Read the model definition and answer for the solid it produces. Units are mm, in the model's axes. Face numbers are marked on the shaded views. Round coordinates to 2 decimals unless told otherwise and drop trailing zeros. Order: outer loops, then holes, each group sorted by start corner. A loop starts at its lowest first (then second) coordinate and runs counter-clockwise, first axis right, second up. Notation, with made-up numbers: (12, 80.5) -> (54, 80.5) arc R13 cw to (54, 89.5) -> close; hole circle Ø7 at (14.25, 28). An arc over 180 degrees is marked (long way). Answer as a JSON object with one key per item and string values. Group by question number.
Item 1: Given P1, Ø4, axis at x = -99, z = 11.5, coming from the +Y side; P2, Ø12, axis at x = 26.5, z = -10, coming from the +Y side; P3, Ø4, axis at x = -99.5, y = 18.5, coming from the +Z side; P4, Ø8, axis at x = -56.5, y = 8, coming from the -Z side, each flat-ended and moving along its own axis, determine where each tip first touches the part or whether it passes through.
Item 2: Section A-A, the plane y = 7 is taken. Write down the section's boundary in (x, z).
Item 3: Consider probe 1 along Z at (x, y) = (-62.5, 6); probe 2 along Y at (x, z) = (50, -9); probe 3 along X at (y, z) = (23.5, -11.5). Determine where each line is inside the solid, lowest interval first. Write a range as from..to.
Item 4: Section D-D, the plane y = 23 is taken. Count the separate pieces of the cut face and the enclosed holes in it, plus the area to 3 significant figures.
Item 5: Section C-C, the plane y = 41.5 is taken. Write down the section's boundary in (x, z).
Item 6: Section B-B, the plane x = -50.5 is taken. Write down the section's boundary in (y, z).
Item 7: The mould has two halves that part along X. Classify the marked faces 1, 2, 3 and 4: pulls with the +X half, pulls with the -X half, needs draft (parallel to the pull), parting line crosses it, or undercut.
from build123d import *

# Parameters (mm, degrees)
ESQUISSE1_W                 = 50
ESQUISSE1_H                 = 50
ESQUISSE1_W_2               = 140
ESQUISSE1_H_2               = 12
BOSS_EXTRU_2_DEPTH          = 12
BOSS_EXTRU_3_DEPTH          = 30
ESQUISSE3_R                 = 4.25
ENL_V_MAT_EXTRU_1_DEPTH     = 110.627399686
ESQUISSE4_R                 = 2.5
ENL_V_MAT_EXTRU_2_DEPTH     = 8
CHANFREIN2_SIZE             = 10
CONG_1_START                = 0.042620229
CONG_1_DEPTH                = 12
BOSS_EXTRU_4_DEPTH          = 40
ENL_V_START                 = -12
ENL_V_MAT_EXTRU_3_OUTLINE_R = 2.5
ENL_V_MAT_EXTRU_3_DEPTH     = 52
ESQUISSE8_R                 = 2.5
ENL_V_MAT_EXTRU_4_DEPTH     = 12


with BuildPart() as part:
    # Esquisse1 → Boss.-Extru.2 (new body)
    with BuildSketch(Plane(origin=(0, 0, 0), x_dir=(1, 0, 0), z_dir=(0, 1, 0))):
        with Locations((69.411764706, -6.042620229)):
            Rectangle(ESQUISSE1_W, ESQUISSE1_H)
        with Locations((-25.588235294, -6.042620229)):
            Rectangle(ESQUISSE1_W_2, ESQUISSE1_H_2)
    extrude(amount=BOSS_EXTRU_2_DEPTH)

    # Esquisse2 → Boss.-Extru.3 (add)
    with BuildSketch(Plane(origin=(0, 0, 0), x_dir=(1, 0, 0), z_dir=(0, 1, 0))):
        Polygon((-95.588235294, -0.042620229), (-95.588235294, 13.957379771), (-103.588235294, 13.957379771), (-103.588235294, -26.042620229), (-95.588235294, -26.042620229), (-95.588235294, -12.042620229), align=None)
    extrude(amount=BOSS_EXTRU_3_DEPTH)

    # Esquisse3 → Enlèv. mat.-Extru.1 (cut, through all)
    with BuildSketch(Plane(origin=(0, 12, 0), x_dir=(1, 0, 0), z_dir=(0, 1, 0))):
        with Locations(Location((69.411764706, -6.042620229, 0), (0, 0, 270))):
            Circle(ESQUISSE3_R)
    extrude(amount=-ENL_V_MAT_EXTRU_1_DEPTH, mode=Mode.SUBTRACT)

    # Esquisse4 → Enlèv. mat.-Extru.2 (cut)
    with BuildSketch(Plane.ZY.offset(103.588235294)):
        with Locations((-6.957379771, 7)):
            Circle(ESQUISSE4_R)
        with Locations((19.042620229, 7)):
            Circle(ESQUISSE4_R)
        with Locations((19.042620229, 23)):
            Circle(ESQUISSE4_R)
        with Locations((-6.957379771, 23)):
            Circle(ESQUISSE4_R)
    extrude(amount=-ENL_V_MAT_EXTRU_2_DEPTH, mode=Mode.SUBTRACT)

    # Chanfrein2
    chanfrein2_edges = [part.edges().sort_by_distance(p)[0] for p in [
        (44.411764706, 6, 31.042620229),
        (44.411764706, 6, -18.957379771),
        (94.411764706, 6, -18.957379771),
    ]]
    chamfer(chanfrein2_edges, length=CHANFREIN2_SIZE)

    # Congé1: read off the stored shape, not the designer's step
    # Congé1 outline → Congé1 (add)
    with BuildSketch(Plane.XY.offset(CONG_1_START)):
        with BuildLine():
            add(Edge.make_bspline(
                [(-95.588235294, 30), (-94.68710818, 12), (-55.638266583, 12)],
                knots=[0, 0, 0, 1, 1, 1], degree=2, weights=[1, 0.724568837, 1]))
            Line((-95.588235294, 30), (-95.588235294, 12))
            Line((-95.588235294, 12), (-55.638266583, 12))
        make_face()
    extrude(amount=CONG_1_DEPTH)

    # Esquisse6 → Boss.-Extru.4 (add)
    with BuildSketch(Plane(origin=(0, 12, 0), x_dir=(1, 0, 0), z_dir=(0, 1, 0))):
        Polygon((94.411764706, -25.042620229), (88.411764706, -31.042620229), (94.411764706, -31.042620229), align=None)
    extrude(amount=BOSS_EXTRU_4_DEPTH)

    # Enlèv. mat.-Extru.3: read off the stored shape, not the designer's step
    # Enlèv. mat.-Extru.3 outline → Enlèv. mat.-Extru.3 (cut)
    with BuildSketch(Plane(origin=(0, 12, 0), x_dir=(1, 0, 0), z_dir=(0, 1, 0)).offset(ENL_V_START)):
        with BuildLine():
            ThreePointArc((94.411764706, -29.042620229), (93.825978268, -30.456833791), (92.411764706, -31.042620229))
            Line((92.411764706, -31.042620229), (94.411764706, -31.042620229))
            Line((94.411764706, -31.042620229), (94.411764706, -29.042620229))
        make_face()
        with Locations((87.411764706, -24.042620229)):
            Circle(ENL_V_MAT_EXTRU_3_OUTLINE_R)
    extrude(amount=ENL_V_MAT_EXTRU_3_DEPTH, mode=Mode.SUBTRACT)

    # Esquisse8 → Enlèv. mat.-Extru.4 (cut)
    with BuildSketch(Plane.XZ):
        with Locations(Location((48.651764706, 6.042620229, 0), (0, 0, 270))):
            Circle(ESQUISSE8_R)
        with Locations(Location((69.411764706, -14.717379771, 0), (0, 0, 270))):
            Circle(ESQUISSE8_R)
    extrude(amount=-ENL_V_MAT_EXTRU_4_DEPTH, mode=Mode.SUBTRACT)


solid = part.part
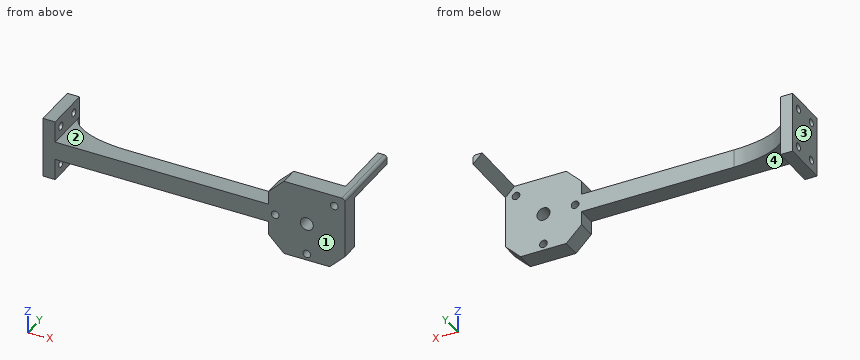
Values found:
{
 "1": {"P1": "y = 30", "P2": "through", "P3": "z = 26.04", "P4": "z = 0.04"},
 "2": {"outline": "(-103.59, -13.96) -> (-95.59, -13.96) -> (-95.59, -9.46) -> (-103.59, -9.46) -> close; (-103.59, -4.46) -> (-95.59, -4.46) -> (-95.59, 0.04) -> (44.41, 0.04) -> (44.41, -8.96) -> (54.41, -18.96) -> (84.41, -18.96) -> (94.41, -8.96) -> (94.41, 29.04) arc R2 ccw to (92.41, 31.04) -> (54.41, 31.04) -> (44.41, 21.04) -> (44.41, 12.04) -> (-95.59, 12.04) -> (-95.59, 16.54) -> (-103.59, 16.54) -> close; (-103.59, 21.54) -> (-95.59, 21.54) -> (-95.59, 26.04) -> (-103.59, 26.04) -> close; hole circle Ø5 at (48.65, 6.04); hole circle Ø8.5 at (69.41, 6.04); hole circle Ø5 at (69.41, -14.72); hole circle Ø5 at (87.41, 24.04)"},
 "3": {"probe 1": "0.04..12.04", "probe 2": "0..12", "probe 3": "-103.59..-95.59"},
 "4": {"separate pieces": "4", "enclosed holes": "0", "area": "297 mm2"},
 "5": {"outline": "(88.41, 31.04) -> (94.41, 25.04) -> (94.41, 29.04) arc R2 ccw to (92.41, 31.04) -> close"},
 "6": {"outline": "(0, 0.04) -> (12, 0.04) -> (12, 12.04) -> (0, 12.04) -> close"},
 "7": {"face 1": "needs draft", "face 2": "undercut", "face 3": "pulls with the -X half", "face 4": "undercut"}
}
